Can you work these out from the model? Positions are in its coordinate system, mm. A direction names the side the tool comes from. Give positions to 0.01 mm unless a question says otherwise; leave off trailing zeros. Order: outer loops, then holes, each group sorted by start corner. A loop starts at its lowest first (then second) coordinate and runs counter-clockwise, first axis right, second up.
```python
from build123d import *

# Parameters (mm, degrees)
F0_W     = 69.342
F0_H     = 140.462
F1_DEPTH = 6.35
F2_T     = -2.54
F4_DEPTH = 25.4
F5_W     = 2.2962929215
F5_H     = 6.5837949514
F5_W_2   = 2.5734174997
F5_H_2   = 7.9922676086
F6_DEPTH = 38.1


with BuildPart() as f1:
    # F0 (on Front) → F1 (new body)
    with BuildSketch(Plane.XZ):
        with Locations((0, 30.688280734)):
            Rectangle(F0_W, F0_H)
    extrude(amount=F1_DEPTH)

    # F2
    f2_openings = [f1.faces().sort_by_distance(p)[0] for p in [
        (0, -6.35, 30.688281),
    ]]
    offset(amount=F2_T, openings=f2_openings)

    # F3 (on face) → F4 (cut)
    with BuildSketch(Plane.XY.offset(100.919280734)):
        with BuildLine():
            ThreePointArc((23.2700649649, -4.7553493267), (22.3264960016, -3.8117803633), (23.2700649649, -2.8682114))
            Line((23.2700649649, -2.8682114), (15.2291525155, -2.8682114))
            ThreePointArc((15.2291525155, -2.8682114), (15.896356528, -3.1445763508), (16.1727214789, -3.8117803633))
            ThreePointArc((16.1727214789, -3.8117803633), (15.896356528, -4.4789843758), (15.2291525155, -4.7553493267))
            Line((15.2291525155, -4.7553493267), (23.2700649649, -4.7553493267))
        make_face()
        with BuildLine():
            ThreePointArc((24.2136339282, -3.8117803633), (23.9372689774, -3.1445763508), (23.2700649649, -2.8682114))
            Line((23.2700649649, -2.8682114), (23.2700649649, -4.7553493267))
            ThreePointArc((23.2700649649, -4.7553493267), (23.9372689774, -4.4789843758), (24.2136339282, -3.8117803633))
        make_face()
        with BuildLine():
            Line((23.2700649649, -4.7553493267), (23.2700649649, -2.8682114))
            ThreePointArc((23.2700649649, -2.8682114), (22.3264960016, -3.8117803633), (23.2700649649, -4.7553493267))
        make_face()
        with BuildLine():
            ThreePointArc((16.1727214789, -3.8117803633), (15.896356528, -3.1445763508), (15.2291525155, -2.8682114))
            Line((15.2291525155, -2.8682114), (15.2291525155, -4.7553493267))
            ThreePointArc((15.2291525155, -4.7553493267), (15.896356528, -4.4789843758), (16.1727214789, -3.8117803633))
        make_face()
        with BuildLine():
            Line((15.2291525155, -4.7553493267), (15.2291525155, -2.8682114))
            ThreePointArc((15.2291525155, -2.8682114), (14.2855835522, -3.8117803633), (15.2291525155, -4.7553493267))
        make_face()
    extrude(amount=-F4_DEPTH, mode=Mode.SUBTRACT)

    # F5 (on Right) → F6 (cut)
    with BuildSketch(Plane.YZ):
        with Locations((-3.7487103837, 90.1714488864)):
            Rectangle(F5_W, F5_H)
        with Locations((-3.9377002977, 80.8853507042)):
            Rectangle(F5_W_2, F5_H_2)
    extrude(amount=-F6_DEPTH, mode=Mode.SUBTRACT)


solid = f1.part
```
1) I'm going to push a flat-ended pin straight in: pin 1 Ø1 at (x, z) = (5.5, 11.5) entering from -Y. Where does the tip first touch, or does it pass through?
2) Suppose I cut it at C-C (z = -19.5). Please give me the cut outline in (x, y), and give its area (3 significant figures).
3) Which directions (+Z, -Z, +X, -X, +Y, -Y) give clear straight access to the entire face, cutting with the end or side of a thin tool? Please do faces 5 (the face through (19, -4.755, 100)), 6 (the face through (0, -3, -39.543)), 7 (the face through (-33, -2.601, 90)), 8 (the face through (-32.131, -4, 30)).
4) If I drill on line 1 (X direction, y = -3.75, z = 9.5); line 2 (Z direction, x = 25.5, y = -3); line 3 (X direction, y = -4.5, z = 84.5), over which ranges is the centre line in solid material (lowest first)?
5) We'd pull the mould along X, two halves only. Please class faces 1 (the face through (0, -3, 100.919)), 2 (the face through (0, -4, -37.003)), 3 (the face through (0, -2.54, 32)), 4 (the face through (-34.671, -3, 30)): +X half, -X half, draft (parallel to the pull), parting line (faces both ways), or undercut.
6) Suppose I cut it at A-A (z = 81). Please give me the cut outline in (x, y), and give its area (3 significant figures).
7) Suppose I cut it at B-B (x = -5.5). Please give me the cut outline in (y, z), and give its area (3 significant figures).
Results:
1. pin 1: stops at y = -2.54
2. outline: (-34.67, -6.35) - (-32.13, -6.35) - (-32.13, -2.54) - (32.13, -2.54) - (32.13, -6.35) - (34.67, -6.35) - (34.67, 0) - (-34.67, 0) - close
2. area: 195 mm2
3. face 5: +Z
3. face 6: -Z, +X, -X, +Y, -Y
3. face 7: -X
3. face 8: -Y
4. line 1: x = -34.67 to -32.13, 32.13 to 34.67
4. line 2: z = -39.54 to -37, 98.38 to 100.92
4. line 3: x = 32.13 to 34.67
5. face 1: draft
5. face 2: undercut
5. face 3: undercut
5. face 4: -X half
6. outline: (-34.67, -6.35) - (-32.13, -6.35) - (-32.13, -5.22) - (-34.67, -5.22) - close; (-34.67, -2.65) - (-32.13, -2.65) - (-32.13, -2.54) - (32.13, -2.54) - (32.13, -6.35) - (34.67, -6.35) - (34.67, 0) - (-34.67, 0) - close
6. area: 189 mm2
7. outline: (-6.35, -39.54) - (0, -39.54) - (0, 100.92) - (-6.35, 100.92) - (-6.35, 98.38) - (-2.54, 98.38) - (-2.54, -37) - (-6.35, -37) - close
7. area: 376 mm2
